from build123d import *

# Parameters (mm, degrees)
SKETCH_1_W          = 42.5
SKETCH_1_H          = 20
EXTRUDE_1_DEPTH     = 20
SKETCH_2_W          = 38.5
SKETCH_2_H          = 20
CUT_EXTRUDE_1_DEPTH = 15
SKETCH_3_R          = 7.25
CUT_EXTRUDE_2_DEPTH = 5
CUT_EXTRUDE_3_REACH = 50.023
SKETCH_4_R          = 1.3
SKETCH_5_R          = 2.1
CUT_EXTRUDE_4_DEPTH = 5
FILLET_1_R          = 4


with BuildPart() as part:
    # 草图1 → 凸台-拉伸1 (new body)
    with BuildSketch(Plane.XY):
        Rectangle(SKETCH_1_W, SKETCH_1_H)
    extrude(amount=EXTRUDE_1_DEPTH)

    # 草图2 → 切除-拉伸1 (cut)
    with BuildSketch(Plane.XY.offset(20)):
        Rectangle(SKETCH_2_W, SKETCH_2_H)
    extrude(amount=-CUT_EXTRUDE_1_DEPTH, mode=Mode.SUBTRACT)

    # 草图3 → 切除-拉伸2 (cut)
    with BuildSketch(Plane(origin=(0, 0, 0), x_dir=(-1, 0, 0), z_dir=(0, 0, -1))):
        Circle(SKETCH_3_R)
    extrude(amount=-CUT_EXTRUDE_2_DEPTH, mode=Mode.SUBTRACT)

    # 切除-拉伸3: up to this face of the body (flat: up to its plane)
    cut_extrude_3_end = Plane(part.part.faces().sort_by_distance((-21.25, 0, 10))[0])
    # 草图4 → 切除-拉伸3 (cut, up to the picked face)
    with BuildSketch(Plane(origin=(21.25, 0, 0), x_dir=(0, 0, -1), z_dir=(1, 0, 0)), mode=Mode.PRIVATE) as cut_extrude_3_sk1:
        with Locations((-17, 0)):
            Circle(SKETCH_4_R)
    cut_extrude_3_tool1 = split(extrude(cut_extrude_3_sk1.sketch, amount=-CUT_EXTRUDE_3_REACH, mode=Mode.PRIVATE), bisect_by=cut_extrude_3_end, keep=Keep.BOTH, mode=Mode.PRIVATE)
    add(cut_extrude_3_tool1.solids().sort_by(Axis((21.25, 0, 17), (-1, 0, 0)))[0], mode=Mode.SUBTRACT)

    # 草图5 → 切除-拉伸4 (cut)
    with BuildSketch(Plane(origin=(0, 0, 0), x_dir=(-1, 0, 0), z_dir=(0, 0, -1))):
        with Locations((-10.5, 0)):
            Circle(SKETCH_5_R)
    extrude(amount=-CUT_EXTRUDE_4_DEPTH, mode=Mode.SUBTRACT)

    # 圆角1
    fillet_1_edges = [part.edges().sort_by_distance(p)[0] for p in [
        (-21.25, 0, 0),
        (21.25, 0, 0),
    ]]
    fillet(fillet_1_edges, radius=FILLET_1_R)


solid = part.part
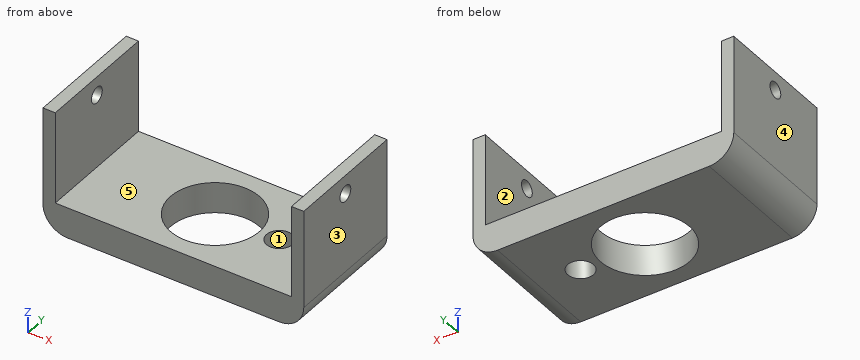
Can you work these out from the model? Positions are in its coordinate system, mm. Face numbers are marked on the shaded views. A direction names the side the tool comes from. Round coordinates to 2 decimals unless told otherwise and drop trailing zeros. Loops run counter-clockwise (first coordinate to the right, second up) from the corner with the lowest first, then second, coordinate; pieces in that order, holes last. Notation, with made-up numbers: (14, 54.5) - (31, 54.5) arc R18 ccw to (31, 74.5) - close; hole circle Ø4 at (49.25, -23.5). An arc over 180 degrees is marked (long way). Answer in a Markdown table with one row per item. Add a question column.
Q1. I want a section at A-A on y = 0. List the corners of the cut face in (x, z) for me.
Q2. I want a section at D-D on z = 13.5. List the corners of the cut face in (x, y) for me, and give its area (3 significant figures).
Q3. For pin 1 Ø10 at (x, y) = (3.5, 3.5) entering from +Z; pin 2 Ø8 at (x, y) = (1.5, 1) entering from -Z; pin 3 Ø5 at (y, z) = (6, 3.5) entering from -X, each with a flat end and sliding along its axis, tell me the tip position at first contact or that it passes through.
Q4. I need wall thicknesses on L1, parallel to X at y = -8.5, z = 9.5; L2, parallel to Z at x = -16.5, y = -5.25; L3, parallel to Y at x = 10.5, z = 3.45. Which ranges of each line are inside material? Lowest first, please.
Q5. We'd pull the mould along X, two halves only. Please class the marked faces 3, 4 and 5: pulls with the +X half, pulls with the -X half, needs draft (parallel to the pull), parting line crosses it, or undercut.
Q6. Which directions (+Z, -Z, +X, -X, +Y, -Y) give clear straight access to the entire face, cutting with the end or side of a thin tool? Please do the marked faces 1 and 2.
Q7. I want a section at B-B on z = 17. List the corners of the cut face in (x, y) for me, and give its area (3 significant figures).
Q8. I want a section at C-C on x = 0. List the corners of the cut face in (y, z) for me.
A:
| question | item | result |
|---|---|---|
| 1 | outline | (-21.25, 4) arc R4 ccw to (-17.25, 0) - (-7.25, 0) - (-7.25, 5) - (-19.25, 5) - (-19.25, 15.7) - (-21.25, 15.7) - close; (-21.25, 18.3) - (-19.25, 18.3) - (-19.25, 20) - (-21.25, 20) - close; (7.25, 0) - (8.4, 0) - (8.4, 5) - (7.25, 5) - close; (12.6, 0) - (17.25, 0) arc R4 ccw to (21.25, 4) - (21.25, 15.7) - (19.25, 15.7) - (19.25, 5) - (12.6, 5) - close; (19.25, 18.3) - (21.25, 18.3) - (21.25, 20) - (19.25, 20) - close |
| 2 | outline | (-21.25, -10) - (-19.25, -10) - (-19.25, 10) - (-21.25, 10) - close; (19.25, -10) - (21.25, -10) - (21.25, 10) - (19.25, 10) - close |
| 2 | area | 80.0 mm^2 |
| 3 | pin 1 | z = 5 |
| 3 | pin 2 | through |
| 3 | pin 3 | x = -21.25 |
| 4 | L1 | -21.25 to -19.25, 19.25 to 21.25 |
| 4 | L2 | 0 to 5 |
| 4 | L3 | -10 to -2.1, 2.1 to 10 |
| 5 | face 3 | pulls with the +X half |
| 5 | face 4 | pulls with the -X half |
| 5 | face 5 | undercut |
| 6 | face 1 | +Z, -Z |
| 6 | face 2 | +Z, +Y, -Y |
| 7 | outline | (-21.25, -10) - (-19.25, -10) - (-19.25, -1.3) - (-21.25, -1.3) - close; (-21.25, 1.3) - (-19.25, 1.3) - (-19.25, 10) - (-21.25, 10) - close; (19.25, -10) - (21.25, -10) - (21.25, -1.3) - (19.25, -1.3) - close; (19.25, 1.3) - (21.25, 1.3) - (21.25, 10) - (19.25, 10) - close |
| 7 | area | 69.6 mm^2 |
| 8 | outline | (-10, 0) - (-7.25, 0) - (-7.25, 5) - (-10, 5) - close; (7.25, 0) - (10, 0) - (10, 5) - (7.25, 5) - close |
